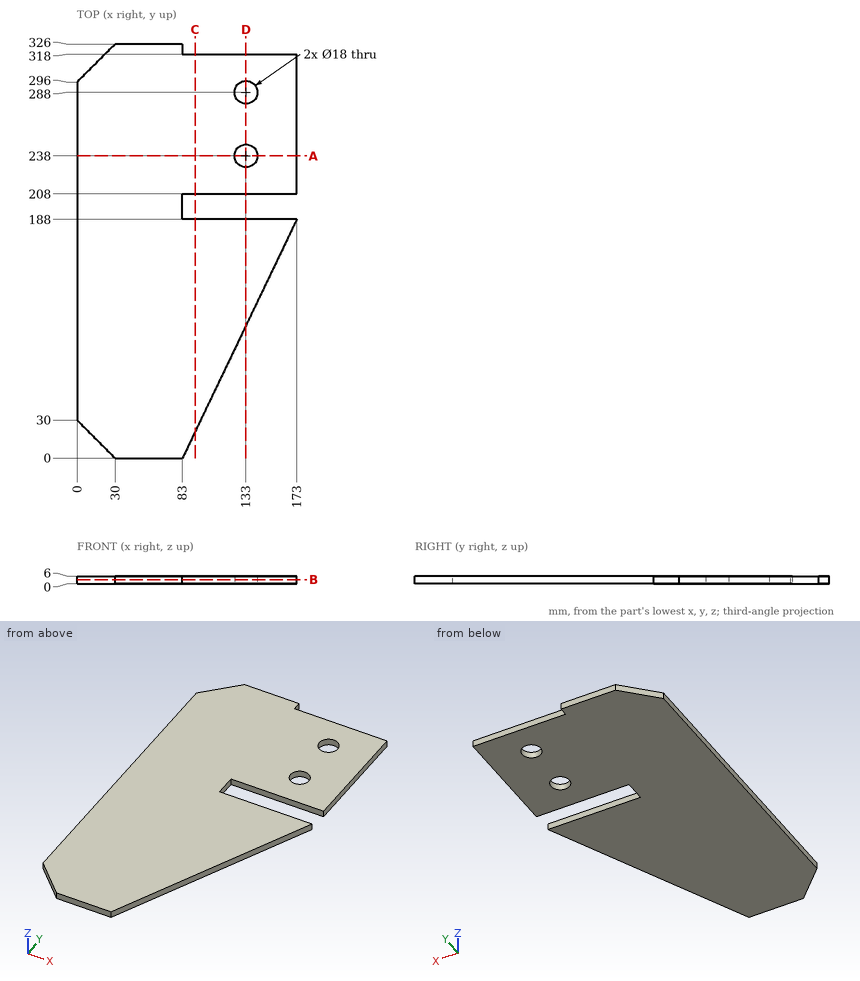
Geometry: see drawing. Coordinates: mm, zero at the bounding-box minimum. Coordinates: 2 decimals unless noted, no trailing zeros. Write each loop counter-clockwise with the first axis right and the second up, starting at its lowest first coordinate (ties: lowest second). Pieces come first, ordered by that corner, then holes. Notation, with made-up numbers: M -0.5,-16 L 51.5,-16 A6 cw 51.5,-8 Z; hole C -34.5,-12 d2. An arc over 180 degrees is marked long. Use CSV: the item, a comma, the result in double quotes. Start each with the question number.
1. Cut plane A-A on y = 238. Return the cut outline in (x, z).
2. Cut plane C-C on x = 93. Return the cut outline in (y, z).
3. Ray query, probe 1 along X at (y, z) = (238, 4.1); probe 2 along Y at (x, z) = (133, 3.55); probe 3 along Y at (x, z) = (137, 5.1). Return the intervals inside material, ascending.
4. Cut plane B-B on z = 3.35. Return the cut outline in (x, y).
5. Cut plane D-D on x = 133. Return the cut outline in (y, z), plus the area to 3 significant figures.
6. First-contact query: P1, Ø3, axis at x = 110, z = 2, coming from the -Y side; P2, Ø11, axis at x = 133, y = 238, coming from the +Z side; P3, Ø3, axis at y = 321.5, z = 3.5, coming from the +X side; P4, Ø1, axis at y = 88.5, z = 4.5, coming from the +X side. Flat tips, straight axial feed; report the tip coordinate or a pass-through.
Entries:
1,outline,"M 0,0 L 124,0 L 124,6 L 0,6 Z; M 142,0 L 173,0 L 173,6 L 142,6 Z"
2,outline,"M 20.89,0 L 188,0 L 188,6 L 20.89,6 Z; M 208,0 L 318,0 L 318,6 L 208,6 Z"
3,probe 1,"0 to 124, 142 to 173"
3,probe 2,"104.44 to 188, 208 to 229, 247 to 279, 297 to 318"
3,probe 3,"112.8 to 188, 208 to 229.94, 246.06 to 279.94, 296.06 to 318"
4,outline,"M 0,30 L 30,0 L 83,0 L 173,188 L 83,188 L 83,208 L 173,208 L 173,318 L 83,318 L 83,326 L 30,326 L 0,296 Z; hole C 133,238 d18; hole C 133,288 d18"
5,outline,"M 104.44,0 L 188,0 L 188,6 L 104.44,6 Z; M 208,0 L 229,0 L 229,6 L 208,6 Z; M 247,0 L 279,0 L 279,6 L 247,6 Z; M 297,0 L 318,0 L 318,6 L 297,6 Z"
5,area,"945 mm²"
6,P1,"y = 53.27"
6,P2,"through"
6,P3,"x = 83"
6,P4,"x = 125.61"
